from build123d import *

# Parameters (mm, degrees)
SKETCH1_W                       = 20
SKETCH1_H                       = 16
BOSS_EXTRUDE1_DEPTH             = 12
SKETCH2_R                       = 3.1
SKETCH2_R_2                     = 1
CUT_EXTRUDE1_DEPTH              = 17
F_2_5_2_5_DIAMETER_HOLE1_D      = 2.5
F_2_5_2_5_DIAMETER_HOLE1_DEPTH  = 4.5
TAP_DRILL_FOR_M6X1_0_TAP1_D     = 5
TAP_DRILL_FOR_M3X0_5_TAP1_D     = 2.5
TAP_DRILL_FOR_M3X0_5_TAP1_DEPTH = 6.999
TAP_DRILL_FOR_M3X0_5_TAP1_TIP   = 0.751075774
CHAMFER1_SIZE                   = 0.5


with BuildPart() as part:
    # Sketch1 → Boss-Extrude1 (new body)
    with BuildSketch(Plane(origin=(0, 0, 0), x_dir=(1, 0, 0), z_dir=(0, 1, 0))):
        Rectangle(SKETCH1_W, SKETCH1_H)
    extrude(amount=BOSS_EXTRUDE1_DEPTH)

    # Sketch2 → Cut-Extrude1 (cut, through all)
    with BuildSketch(Plane.XY.offset(8)):
        with Locations((1, 7)):
            Circle(SKETCH2_R)
        with Locations((3, 2)):
            Circle(SKETCH2_R_2)
    extrude(amount=-CUT_EXTRUDE1_DEPTH, mode=Mode.SUBTRACT)

    # Ø2.5 (2.5) Diameter Hole1
    with Locations(Plane.XY.offset(8)):
        with Locations((-8, 2)):
            Hole(F_2_5_2_5_DIAMETER_HOLE1_D / 2, depth=F_2_5_2_5_DIAMETER_HOLE1_DEPTH)

    # Tap Drill for M6x1.0 Tap1 (through all)
    with Locations(Plane(origin=(0, 12, 0), x_dir=(1, 0, 0), z_dir=(0, 1, 0))):
        with Locations((-6, 0)):
            Hole(TAP_DRILL_FOR_M6X1_0_TAP1_D / 2)

    # Tap Drill for M3x0.5 Tap1
    with Locations(Plane(origin=(0, 0, 0), x_dir=(-1, 0, 0), z_dir=(0, -1, 0))):
        with Locations((0, 0)):
            Hole(TAP_DRILL_FOR_M3X0_5_TAP1_D / 2, depth=TAP_DRILL_FOR_M3X0_5_TAP1_DEPTH)
            with Locations((0, 0, -(TAP_DRILL_FOR_M3X0_5_TAP1_DEPTH + TAP_DRILL_FOR_M3X0_5_TAP1_TIP / 2))):  # 118° drill point
                Cone(0, TAP_DRILL_FOR_M3X0_5_TAP1_D / 2, TAP_DRILL_FOR_M3X0_5_TAP1_TIP, mode=Mode.SUBTRACT)

    # Chamfer1
    chamfer1_edges = [part.edges().sort_by_distance(p)[0] for p in [
        (0, 12, -8),
        (-10, 12, 0),
        (-3.5, 12, 0),
        (-3.5, 0, 0),
        (-1.25, 0, 0),
        (0, 12, 8),
        (-10, 0, 0),
        (0, 0, -8),
        (10, 0, 0),
        (0, 0, 8),
        (10, 12, 0),
        (-10, 6, 8),
        (-10, 6, -8),
        (10, 6, -8),
        (10, 6, 8),
    ]]
    chamfer(chamfer1_edges, length=CHAMFER1_SIZE)


solid = part.part
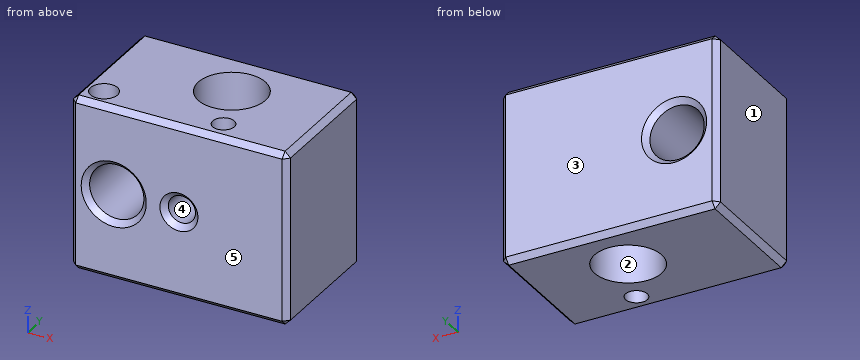
Design review of the part built by this model. Coordinates are the model's own, in mm. Face numbers are marked on the shaded views. A direction names the side the tool comes from. Coordinates: 2 decimals unless noted, no trailing zeros. Loops run counter-clockwise (first coordinate to the right, second up) from the corner with the lowest first, then second, coordinate; pieces in that order, holes last.
Item 1: For the marked faces 4 and 5, list the 3-axis set-ups (+Z, -Z, +X, -X, +Y, -Y) from which the entire face can be reached by the end or side of a thin tool; tool diameter is ignored.
Completed:
face 4: -Y
face 5: +Z, -Z, +X, -X, -Y
Item 2: Add section D-D (x = -6). Write out the cut boundary in (y, z), and give its area (3 significant figures).
Completed:
outline: (0, -7.5) - (0.5, -8) - (11.5, -8) - (12, -7.5) - (12, -3) - (11.5, -2.5) - (0.5, -2.5) - (0, -3) - close; (0, 3) - (0.5, 2.5) - (11.5, 2.5) - (12, 3) - (12, 7.5) - (11.5, 8) - (0.5, 8) - (0, 7.5) - close
area: 131 mm2
Item 3: Draft analysis for pull direction Y (two halves, no side actions). For the marked faces 1, 2 and 3, state which applies: pulls with the +Y half, pulls with the -Y half, needs draft (parallel to the pull), parting line crosses it, or undercut.
Completed:
face 1: needs draft
face 2: undercut
face 3: pulls with the +Y half
Item 4: Add section A-A (y = 2). Write out the cut boundary in (x, z).
Completed:
outline: (-10, -7.5) - (-9.5, -8) - (2, -8) - (2, 8) - (-6.75, 8) - (-6.75, 3.5) - (-9.25, 3.5) - (-9.25, 8) - (-9.5, 8) - (-10, 7.5) - close; (4, -8) - (9.5, -8) - (10, -7.5) - (10, 7.5) - (9.5, 8) - (4, 8) - close; hole circle Ø5 at (-6, 0); hole circle Ø2.5 at (0, 0)
Item 5: Wall thickness on L1, parallel to Y at x = -8, z = 5.15; L2, parallel to X at y = 8, z = 0.5; L3, parallel to X at y = 6.75, z = 0: over which ranges is each line inside the solid? List them lowest first.
Completed:
L1: y = 0 to 0.75, 3.25 to 12
L2: x = -10 to -8.45, -3.55 to -1.93, 3.93 to 10
L3: x = -10 to -8.5, -3.5 to -2.09, 4.09 to 10
Item 6: Add section B-B (y = 6.75). Write out the cut boundary in (x, z), and give its area (3 significant figures).
Completed:
outline: (-10, -7.5) - (-9.5, -8) - (-2.09, -8) - (-2.09, 8) - (-9.5, 8) - (-10, 7.5) - close; (4.09, -8) - (9.5, -8) - (10, -7.5) - (10, 7.5) - (9.5, 8) - (4.09, 8) - close; hole circle Ø5 at (-6, 0)
area: 201 mm2
Item 7: Add section C-C (z = 5.25). Write out the cut boundary in (x, y), and give its area (3 significant figures).
Completed:
outline: (-10, 0.5) - (-9.5, 0) - (9.5, 0) - (10, 0.5) - (10, 11.5) - (9.5, 12) - (-9.5, 12) - (-10, 11.5) - close; hole circle Ø2.5 at (-8, 2); hole circle Ø6.2 at (1, 7); hole circle Ø2 at (3, 2)
area: 201 mm2
